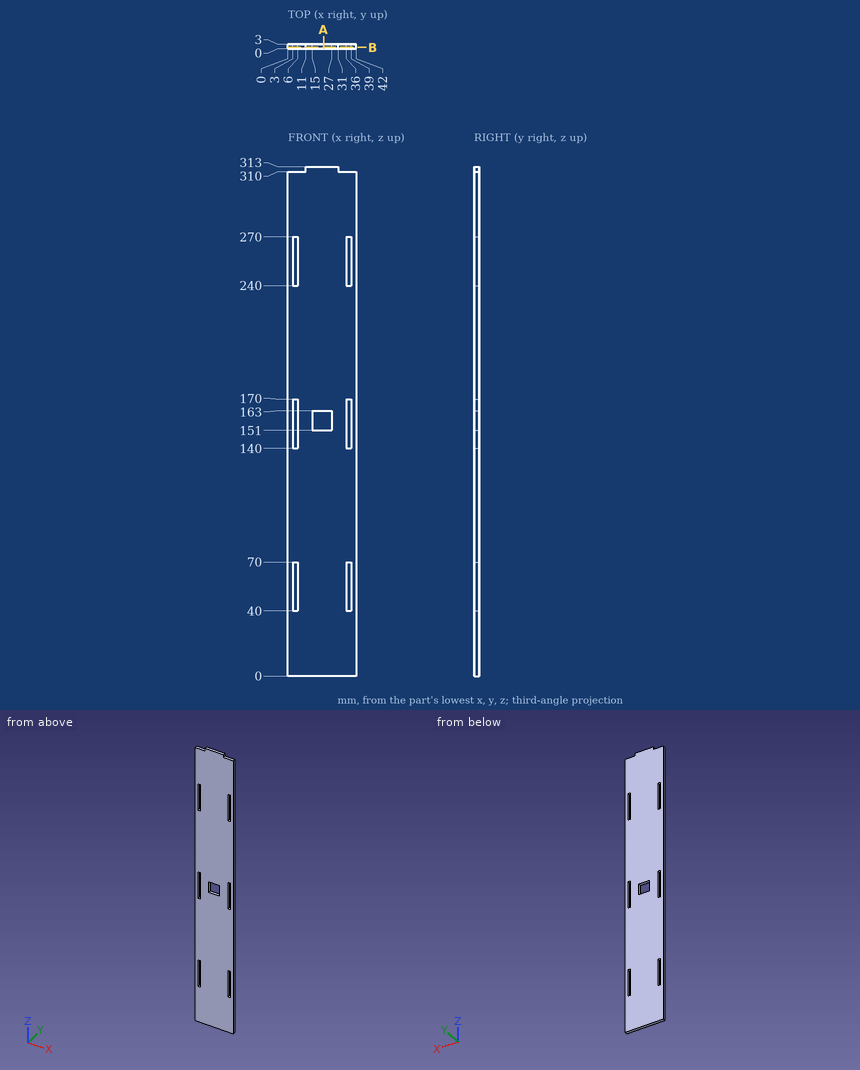
Verification items for this drawing (mm, ordinates from the low corner). Give positions to 0.01 mm unless a question says otherwise; leave off trailing zeros. Loops run counter-clockwise (first coordinate to the right, second up) from the corner with the lowest first, then second, coordinate; pieces in that order, holes last. Notation, with made-up numbers: M 29.25,-32 L 66.25,-32 A21 cw 66.25,-9 Z; hole C 45.25,1 d6. An arc over 180 degrees is marked long. Return JSON: item names as keys, results as strings. Group by question number.
1. Cross-section at B-B on y = 0.95. State how many separate pieces and enclosed holes the cut face has, plus the area to 3 significant figures.
2. Go/stop test with flat-tipped pins: pin 1 (1.5 mm diameter, centred on x = 37, y = 1, fed in from +Z); pin 2 (1.5 mm diameter, centred on y = 2, z = 311, fed in from -X). Record where each tip stops, or that it passes through.
3. Thickness scan on L1, parallel to Z at x = 5, y = 0.7; L2, parallel to X at y = 2.3, z = 155; L3, parallel to Z at x = 20, y = 0.2. Record the ranges inside material, lowest first.
4. Cross-section at A-A on x = 22. Record the boundary of the cut face in (y, z), plus the area to 3 significant figures.
Return value:
{
 "1": {"separate pieces": "1", "enclosed holes": "7", "area": "12,400 mm^2"},
 "2": {"pin 1": "z = 310", "pin 2": "x = 11"},
 "3": {"L1": "0 to 40, 70 to 140, 170 to 240, 270 to 310", "L2": "0 to 3, 6 to 15, 27 to 36, 39 to 42", "L3": "0 to 151, 163 to 313"},
 "4": {"outline": "M 0,0 L 3,0 L 3,151 L 0,151 Z; M 0,163 L 3,163 L 3,313 L 0,313 Z", "area": "903 mm^2"}
}
